Autodesk Inventor part; units mm, degrees
ref_plane "YZ Plane" through (0, 0, 0) normal (1, 0, 0) x (0, 1, 0)
ref_plane "XZ Plane" through (0, 0, 0) normal (0, 1, 0) x (-1, 0, 0)
ref_plane "XY Plane" through (0, 0, 0) normal (0, 0, 1) x (1, 0, 0)
sketch "Sketch9" plane through (0, 0, 0) normal (0, 1, 0) x (-1, 0, 0)
  line L0 (15, 15) -> (-15, 15)
  line L1 (-15, 15) -> (-15, -15)
  line L2 (-15, -15) -> (15, -15)
  line L3 (15, -15) -> (15, 15)
  line L4 (15, 15) -> (-15, -15) construction
  line L5 (-15, 15) -> (15, -15) construction
  line L6 (-13, 13) -> (13, 13)
  line L7 (13, 13) -> (13, -13)
  line L8 (13, -13) -> (-13, -13)
  line L9 (-13, -13) -> (-13, 13)
  point P0 (0, 0)
  dimension "d172" = 30
  dimension "d173" = 30
  dimension "d174" = 2
extrude "Extrusion3" add sketch "Sketch9" against normal blind 130
sketch "Sketch10" plane through (0, 0, 0) normal (1, 0, 0) x (0, 1, 0)
  line L0 (0, 15) -> (0, -15) construction
  line L1 (0, 15) -> (-130, 15) construction
  line L2 (-130, -15) -> (-130, 15) construction
  line L3 (0, -15) -> (-130, -15) construction
  line L4 (-58.5, 8.5) -> (-41.5, 8.5)
  line L5 (-41.5, 8.5) -> (-41.5, -8.5)
  line L6 (-41.5, -8.5) -> (-58.5, -8.5)
  line L7 (-58.5, -8.5) -> (-58.5, 8.5)
  line L8 (-58.5, 8.5) -> (-41.5, -8.5) construction
  line L9 (-41.5, 8.5) -> (-58.5, -8.5) construction
  line L10 (0, 0) -> (30, 0)
  circle A0 centre (-50, 0) radius 8.5
  dimension "d177" = 17
  dimension "d178" = 17
  dimension "d181" = 30
  dimension "d182" = 80
extrude "Extrusion4" cut sketch "Sketch10" along normal through all contours A0
pattern_linear "Rectangular Pattern4" count 2 spacing 55 along (0, -1, 0) of "Extrusion4"
properties part number "PRS 1200-54-01 FDS 1200 way tube 3" material "Stainless Steel"
Could you check a few things on this model? Use its own coordinates, in mm. A direction names the side the tool comes from. Coordinates: 2 decimals unless noted, no trailing zeros. Write each loop counter-clockwise with the first axis right and the second up, starting at its lowest first coordinate (ties: lowest second). Pieces come first, ordered by that corner, then holes. Notation, with made-up numbers: (61.25, 73) - (84.25, 73) arc R24 ccw to (84.25, 89) - close; hole circle Ø10 at (11.25, 24.25). An arc over 180 degrees is marked (long way). Use a Markdown table: item, result.
Q1. I'm going to push a flat-ended pin straight in: pin 1 Ø3 at (x, z) = (10.5, 6) entering from +Y. Where does the tip first touch, or does it pass through?
Geometry check:
| item | result |
|---|---|
| pin 1 | passes through |
Q2. Imagine slicing it at D-D (z = -1.75). List the corners of the cut face in (x, y) for me, and give its area (3 significant figures).
Geometry check:
| item | result |
|---|---|
| outline | (-15, -130) - (-13, -130) - (-13, 0) - (-15, 0) - close; (13, -130) - (15, -130) - (15, -113.32) - (13, -113.32) - close; (13, -96.68) - (15, -96.68) - (15, -58.32) - (13, -58.32) - close; (13, -41.68) - (15, -41.68) - (15, 0) - (13, 0) - close |
| area | 453 mm2 |
Q3. Imagine slicing it at C-C (y = -46). List the corners of the cut face in (x, z) for me.
Geometry check:
| item | result |
|---|---|
| outline | (-15, -15) - (15, -15) - (15, -7.5) - (13, -7.5) - (13, -13) - (-13, -13) - (-13, 13) - (13, 13) - (13, 7.5) - (15, 7.5) - (15, 15) - (-15, 15) - close |
Q4. Imagine slicing it at A-A (x = 1.25). List the corners of the cut face in (y, z) for me.
Geometry check:
| item | result |
|---|---|
| outline | (-130, -15) - (0, -15) - (0, -13) - (-130, -13) - close; (-130, 13) - (0, 13) - (0, 15) - (-130, 15) - close |
Q5. Thinking about a two-plate mould opening in Z: for faces 4 (the flat face through (0, -64, -15)), 5 (the flat face through (-15, -64, 0)), 6 (the cylindrical face through (13.99, -113.49, -0.37)), 7 (the flat face through (0, -64, 15)), which applies, +Z half, -Z half, draft (parallel to the pull), parting line (faces both ways), or undercut?
Geometry check:
| item | result |
|---|---|
| face 4 | -Z half |
| face 5 | draft |
| face 6 | undercut |
| face 7 | +Z half |
Q6. Imagine slicing it at B-B (z = 9.75). List the corners of the cut face in (x, y) for me.
Geometry check:
| item | result |
|---|---|
| outline | (-15, -130) - (-13, -130) - (-13, 0) - (-15, 0) - close; (13, -130) - (15, -130) - (15, 0) - (13, 0) - close |
Q7. Please list where these lines run through material, in increasing order: L1, parallel to Y at x = 14.15, z = 0; L2, parallel to X at y = -42, z = 9.25.
Geometry check:
| item | result |
|---|---|
| L1 | y = -130 to -113.5, -96.5 to -58.5, -41.5 to 0 |
| L2 | x = -15 to -13, 13 to 15 |
Q8. Which directions (+Z, -Z, +X, -X, +Y, -Y) give clear straight access to the entire face, cutting with the end or side of a thin tool? Please do faces 1 (the flat face through (13, -64, 0)), 2 (the cylindrical face through (13.986, -56.265, -5.745)), 3 (the flat face through (15, -64, 0)).
Geometry check:
| item | result |
|---|---|
| face 1 | +Y, -Y |
| face 2 | +X |
| face 3 | +Z, -Z, +X, +Y, -Y |
